Geometry: see drawing. Coordinates: mm, zero at the bounding-box minimum. Round coordinates to 2 decimals unless told otherwise and drop trailing zeros. Loops run counter-clockwise (first coordinate to the right, second up) from the corner with the lowest first, then second, coordinate; pieces in that order, holes last.
(1) Section D-D, the plane z = 2.9. Return the cut outline in (x, y) (3 decimals).
(2) Mould query, pull axis X, two halves, no side actions, for the marked faces 1, 2 and 3. Classes: pulls with the +X half, pulls with the -X half, needs draft (parallel to the pull), parting line crosses it, or undercut.
(3) First-contact query: pin 1 Ø2.5 at (x, y) = (24, 3) entering from -Z; pin 2 Ø3 at (x, z) = (5, 2.5) entering from -Y. Flat tips, straight axial feed; report the tip coordinate or a pass-through.
(4) Section B-B, the plane x = 24. Return the cut outline in (y, z) (3 decimals), plus the area to 3 significant figures.
(5) Material intervals for probe 1 along X at (y, z) = (2.7, 0.95); probe 2 along X at (y, z) = (2.65, 3); probe 3 along X at (y, z) = (3.95, 5.3), sorted ascending.
(6) Section A-A, the plane z = 0.9. Return the cut outline in (x, y) (3 decimals), plus the area to 3 significant figures.
(7) Section C-C, the plane y = 4.05. Return the cut outline in (x, z).
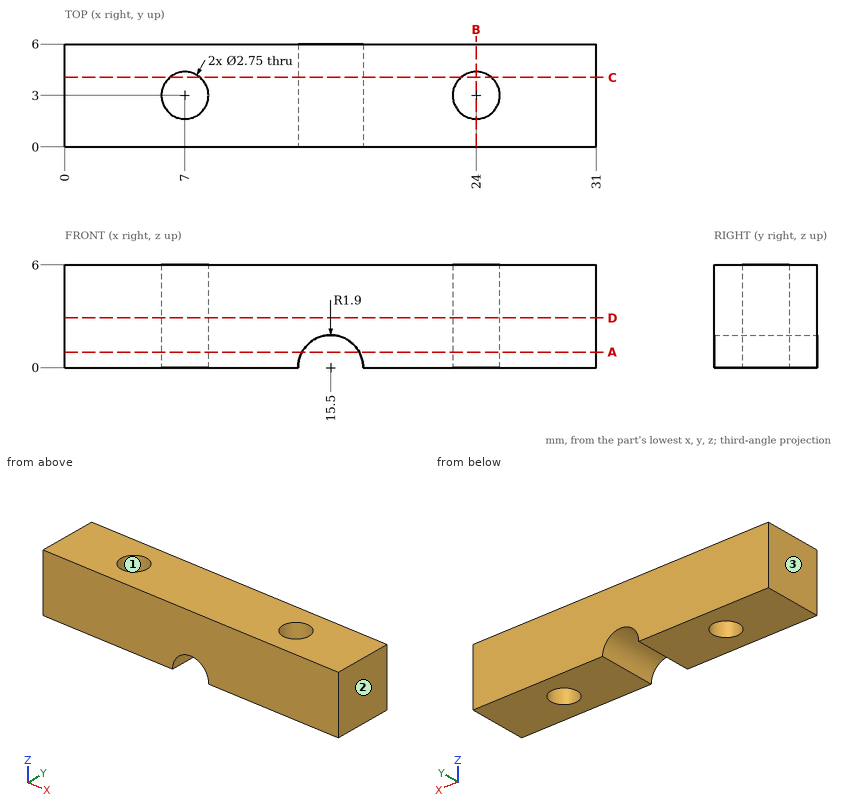
Output values:
1. outline: (0, 0) - (31, 0) - (31, 6) - (0, 6) - close; hole circle Ø2.75 at (7, 3); hole circle Ø2.75 at (24, 3)
2. face 1: undercut
2. face 2: pulls with the +X half
2. face 3: pulls with the -X half
3. pin 1: passes through
3. pin 2: stops at y = 0
4. outline: (0, 0) - (1.625, 0) - (1.625, 6) - (0, 6) - close; (4.375, 0) - (6, 0) - (6, 6) - (4.375, 6) - close
4. area: 19.5 mm2
5. probe 1: x = 0 to 5.66, 8.34 to 13.85, 17.15 to 22.66, 25.34 to 31
5. probe 2: x = 0 to 5.67, 8.33 to 22.67, 25.33 to 31
5. probe 3: x = 0 to 6.01, 7.99 to 23.01, 24.99 to 31
6. outline: (0, 0) - (13.827, 0) - (13.827, 6) - (0, 6) - close; (17.173, 0) - (31, 0) - (31, 6) - (17.173, 6) - close; hole circle Ø2.75 at (7, 3); hole circle Ø2.75 at (24, 3)
6. area: 154 mm2
7. outline: (0, 0) - (6.11, 0) - (6.11, 6) - (0, 6) - close; (7.89, 0) - (13.6, 0) arc R1.9 cw to (17.4, 0) - (23.11, 0) - (23.11, 6) - (7.89, 6) - close; (24.89, 0) - (31, 0) - (31, 6) - (24.89, 6) - close
